```python
from build123d import *

# Parameters (mm, degrees)
SKETCH047_W              = 20.32
SKETCH047_H              = 15.24
PAD001010_DEPTH          = 1.65
SKETCH048_R              = 0.39
POCKET021005005004_DEPTH = 1.651
LINEARPATTERN002_COUNT   = 8
LINEARPATTERN002_PITCH   = 2.54


with BuildPart() as part:
    # Sketch047 → Pad001010 (new body)
    with BuildSketch(Plane.XY):
        Rectangle(SKETCH047_W, SKETCH047_H)
    extrude(amount=PAD001010_DEPTH)

    # Sketch048 (on Face6 of Pad001010) → Pocket021005005004 (cut, through all)
    with BuildSketch(Plane.XY.offset(1.65)):
        with Locations((-8.89, -6.35)):
            Circle(SKETCH048_R)
        with Locations((-8.89, 6.35)):
            Circle(SKETCH048_R)
    pocket021005005004 = extrude(amount=-POCKET021005005004_DEPTH, mode=Mode.SUBTRACT)

    # LinearPattern002: Pocket021005005004 ×8
    with Locations(*[(i * LINEARPATTERN002_PITCH, 0, 0) for i in range(1, LINEARPATTERN002_COUNT)]):
        add(pocket021005005004, mode=Mode.SUBTRACT)


solid = part.part
```
Build history of the part. All positions in model axes, mm. Coordinates: 2 decimals unless noted, no trailing zeros. Write each loop counter-clockwise with the first axis right and the second up, starting at its lowest first coordinate (ties: lowest second). Pieces come first, ordered by that corner, then holes.
1. Band-saw the part on B-B, the plane z = 0.65. Give the number of separate pieces and of enclosed holes in the cut face, and give its area (3 significant figures).
Answer block:
separate pieces: 1
enclosed holes: 16
area: 302 mm2
2. Band-saw the part on A-A, the plane x = -6.35. Give the cut face in (y, z).
Answer block:
outline: (-7.62, 0) - (-6.74, 0) - (-6.74, 1.65) - (-7.62, 1.65) - close; (-5.96, 0) - (5.96, 0) - (5.96, 1.65) - (-5.96, 1.65) - close; (6.74, 0) - (7.62, 0) - (7.62, 1.65) - (6.74, 1.65) - close
3. Drill centre lines: probe 1 along Y at (x, z) = (3.81, 1.3); probe 2 along Y at (x, z) = (1, 0.85). Where is each one in solid material? Low to high.
Answer block:
probe 1: y = -7.62 to -6.74, -5.96 to 5.96, 6.74 to 7.62
probe 2: y = -7.62 to -6.63, -6.07 to 6.07, 6.63 to 7.62
